Design review of the part built by this model. Coordinates are the model's own, in mm. Give positions to 0.01 mm unless a question says otherwise; leave off trailing zeros. Loops run counter-clockwise (first coordinate to the right, second up) from the corner with the lowest first, then second, coordinate; pieces in that order, holes last. Notation, with made-up numbers: (-19, -2) - (20, -2) arc R7 cw to (20, 5) - close; hole circle Ø3 at (40, -23). An arc over 180 degrees is marked (long way). Write each question's results on one line, items separated by ' | '.
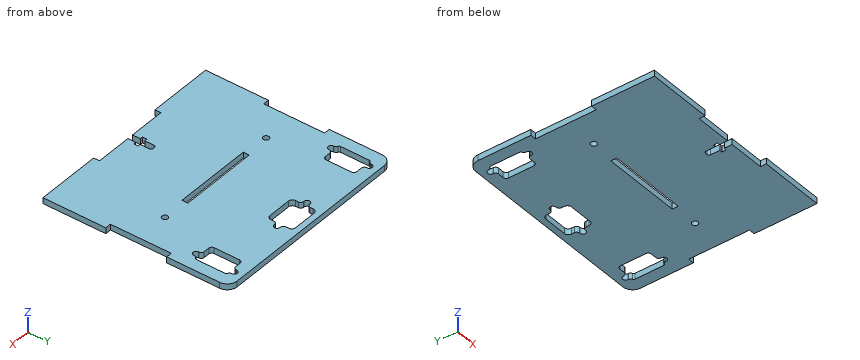
from build123d import *

# Parameters (mm, degrees)
ESBO_O1_W                = 100
ESBO_O1_H                = 95
RESSALTO_EXTRUS_O1_DEPTH = 1.5
ESBO_O2_R                = 1.5
ESBO_O2_W                = 40
ESBO_O2_H                = 3
CORTE_EXTRUS_O1_DEPTH    = 70.030790232
ESBO_O3_W                = 3
ESBO_O3_H                = 32
RESSALTO_EXTRUS_O2_DEPTH = 3
CUT_EXTRUDE1_DEPTH       = 72.233770081
CUT_EXTRUDE1_DEPTH_BACK  = 72.233770081
CUT_EXTRUDE4_DEPTH       = 72.186375101
CUT_EXTRUDE4_DEPTH_BACK  = 72.186375101
FILLET1_R                = 5


with BuildPart() as part:
    # Esboço1 → Ressalto-extrusão1 (new, symmetric)
    with BuildSketch(Plane.XY):
        Rectangle(ESBO_O1_W, ESBO_O1_H)
    extrude(amount=RESSALTO_EXTRUS_O1_DEPTH, both=True)

    # Esboço2 → Corte-extrusão1 (cut, through all)
    with BuildSketch(Plane.XY.offset(1.5)):
        with Locations((-33, -1)):
            Circle(ESBO_O2_R)
        with Locations(Location((33, -1, 0), (0, 0, 180))):
            Circle(ESBO_O2_R)
        with Locations((0, -46)):
            Rectangle(ESBO_O2_W, ESBO_O2_H)
        with Locations((0, -1)):
            Rectangle(ESBO_O2_W, ESBO_O2_H)
    extrude(amount=-CORTE_EXTRUS_O1_DEPTH, mode=Mode.SUBTRACT)

    # Esboço3 → Ressalto-extrusão2 (add, through all)
    with BuildSketch(Plane.XY.offset(1.5)):
        with Locations((-51.5, -31.5)):
            Rectangle(ESBO_O3_W, ESBO_O3_H)
        with Locations((51.5, -31.5)):
            Rectangle(ESBO_O3_W, ESBO_O3_H)
        with Locations((-51.5, 31.5)):
            Rectangle(ESBO_O3_W, ESBO_O3_H)
        with Locations((51.5, 31.5)):
            Rectangle(ESBO_O3_W, ESBO_O3_H)
    extrude(amount=-RESSALTO_EXTRUS_O2_DEPTH)

    # Sketch1 → Cut-Extrude1 (cut, two sides: drawn at the far end of the back side and taken through both)
    with BuildSketch(Plane(origin=(0, 0, -1.5), x_dir=(-1, 0, 0), z_dir=(0, 0, -1)).offset(-CUT_EXTRUDE1_DEPTH_BACK)):
        with BuildLine():
            Line((-36.5, 39.75), (-36.5, 26.75))
            ThreePointArc((-36.5, 26.75), (-36.939339828, 25.689339828), (-38, 25.25))
            Line((-38, 25.25), (-41, 25.25))
            ThreePointArc((-41, 25.25), (-42.060660172, 24.810660172), (-42.5, 23.75))
            Line((-42.5, 23.75), (-42.5, 23.5))
            ThreePointArc((-42.5, 23.5), (-44, 22), (-45.5, 23.5))
            Line((-45.5, 23.5), (-45.5, 23.75))
            ThreePointArc((-45.5, 23.75), (-45.74500996, 24.571583836), (-46.4, 25.124772708))
            ThreePointArc((-46.4, 25.124772708), (-46.836660027, 25.49356529), (-47, 26.041287847))
            Line((-47, 26.041287847), (-47, 40.458712153))
            ThreePointArc((-47, 40.458712153), (-46.836660027, 41.00643471), (-46.4, 41.375227292))
            ThreePointArc((-46.4, 41.375227292), (-45.74500996, 41.928416164), (-45.5, 42.75))
            Line((-45.5, 42.75), (-45.5, 43))
            ThreePointArc((-45.5, 43), (-44, 44.5), (-42.5, 43))
            Line((-42.5, 43), (-42.5, 42.75))
            ThreePointArc((-42.5, 42.75), (-42.060660172, 41.689339828), (-41, 41.25))
            Line((-41, 41.25), (-38, 41.25))
            ThreePointArc((-38, 41.25), (-36.939339828, 40.810660172), (-36.5, 39.75))
        make_face()
        with BuildLine():
            Line((-6, 44.5), (6, 44.5))
            ThreePointArc((6, 44.5), (7.414213562, 43.914213562), (8, 42.5))
            Line((8, 42.5), (8, 41))
            ThreePointArc((8, 41), (8.439339828, 39.939339828), (9.5, 39.5))
            Line((9.5, 39.5), (9.75, 39.5))
            ThreePointArc((9.75, 39.5), (11.25, 38), (9.75, 36.5))
            Line((9.75, 36.5), (9.5, 36.5))
            ThreePointArc((9.5, 36.5), (8.439339828, 36.060660172), (8, 35))
            Line((8, 35), (8, 33.5))
            ThreePointArc((8, 33.5), (7.414213562, 32.085786438), (6, 31.5))
            Line((6, 31.5), (-6, 31.5))
            ThreePointArc((-6, 31.5), (-7.414213562, 32.085786438), (-8, 33.5))
            Line((-8, 33.5), (-8, 35))
            ThreePointArc((-8, 35), (-8.439339828, 36.060660172), (-9.5, 36.5))
            Line((-9.5, 36.5), (-9.75, 36.5))
            ThreePointArc((-9.75, 36.5), (-11.25, 38), (-9.75, 39.5))
            Line((-9.75, 39.5), (-9.5, 39.5))
            ThreePointArc((-9.5, 39.5), (-8.439339828, 39.939339828), (-8, 41))
            Line((-8, 41), (-8, 42.5))
            ThreePointArc((-8, 42.5), (-7.414213562, 43.914213562), (-6, 44.5))
        make_face()
        with BuildLine():
            Line((47, 40.458712153), (47, 26.041287847))
            ThreePointArc((47, 26.041287847), (46.836660027, 25.49356529), (46.4, 25.124772708))
            ThreePointArc((46.4, 25.124772708), (45.74500996, 24.571583836), (45.5, 23.75))
            Line((45.5, 23.75), (45.5, 23.5))
            ThreePointArc((45.5, 23.5), (44, 22), (42.5, 23.5))
            Line((42.5, 23.5), (42.5, 23.75))
            ThreePointArc((42.5, 23.75), (42.060660172, 24.810660172), (41, 25.25))
            Line((41, 25.25), (38, 25.25))
            ThreePointArc((38, 25.25), (36.939339828, 25.689339828), (36.5, 26.75))
            Line((36.5, 26.75), (36.5, 39.75))
            ThreePointArc((36.5, 39.75), (36.939339828, 40.810660172), (38, 41.25))
            Line((38, 41.25), (41, 41.25))
            ThreePointArc((41, 41.25), (42.060660172, 41.689339828), (42.5, 42.75))
            Line((42.5, 42.75), (42.5, 43))
            ThreePointArc((42.5, 43), (44, 44.5), (45.5, 43))
            Line((45.5, 43), (45.5, 42.75))
            ThreePointArc((45.5, 42.75), (45.74500996, 41.928416164), (46.4, 41.375227292))
            ThreePointArc((46.4, 41.375227292), (46.836660027, 41.00643471), (47, 40.458712153))
        make_face()
    extrude(amount=CUT_EXTRUDE1_DEPTH + CUT_EXTRUDE1_DEPTH_BACK, mode=Mode.SUBTRACT)

    # Sketch2 → Cut-Extrude4 (cut, two sides: drawn at the far end of the back side and taken through both)
    with BuildSketch(Plane.XY.offset(-CUT_EXTRUDE4_DEPTH_BACK)):
        with BuildLine():
            Line((-0.5, -32.5), (0.5, -32.5))
            ThreePointArc((0.5, -32.5), (1.207106781, -32.792893219), (1.5, -33.5))
            Line((1.5, -33.5), (1.5, -38.23))
            Line((1.5, -38.23), (2.85, -38.23))
            Line((2.85, -38.23), (2.85, -40.5))
            Line((2.85, -40.5), (1.5, -40.5))
            Line((1.5, -40.5), (1.5, -44.5))
            Line((1.5, -44.5), (-1.5, -44.5))
            Line((-1.5, -44.5), (-1.5, -40.5))
            Line((-1.5, -40.5), (-2.85, -40.5))
            Line((-2.85, -40.5), (-2.85, -38.23))
            Line((-2.85, -38.23), (-1.5, -38.23))
            Line((-1.5, -38.23), (-1.5, -33.5))
            ThreePointArc((-1.5, -33.5), (-1.207106781, -32.792893219), (-0.5, -32.5))
        make_face()
    extrude(amount=CUT_EXTRUDE4_DEPTH + CUT_EXTRUDE4_DEPTH_BACK, mode=Mode.SUBTRACT)

    # Fillet1
    fillet1_edges = [part.edges().sort_by_distance(p)[0] for p in [
        (53, 47.5, 0),
        (-53, 47.5, 0),
    ]]
    fillet(fillet1_edges, radius=FILLET1_R)


solid = part.part
(1) Take a section at D-D on x = 15.5. Give the boundary of the cut face in (y, z), plus the area to 3 significant figures.
Answers below:
outline: (-44.5, -1.5) - (-2.5, -1.5) - (-2.5, 1.5) - (-44.5, 1.5) - close; (0.5, -1.5) - (47.5, -1.5) - (47.5, 1.5) - (0.5, 1.5) - close | area: 267 mm2
(2) Take a section at C-C on y = 13.5. Give the boundary of the cut face in (x, z), plus the area to 3 significant figures.
Answers below:
outline: (-50, -1.5) - (50, -1.5) - (50, 1.5) - (-50, 1.5) - close | area: 300 mm2
(3) Take a section at B-B on z = 0.2. Count the separate pieces of the cut face and the enclosed holes in it, plus the area to 3 significant figures.
Answers below:
separate pieces: 1 | enclosed holes: 6 | area: 8,980 mm2
(4) Take a section at A-A on x = 44. Give the boundary of the cut face in (y, z).
Answers below:
outline: (-47.5, -1.5) - (22, -1.5) - (22, 1.5) - (-47.5, 1.5) - close; (44.5, -1.5) - (47.5, -1.5) - (47.5, 1.5) - (44.5, 1.5) - close
(5) Wall thickness on line 1 along Y through (x, z) = (4, 0.45); line 2 along Y through (x, z) = (-0.5, -1.05); line 3 along Y through (x, z) = (33, -0.1): over which ranges is each line inside the solid? List them lowest first. Write a range as from..to.
Answers below:
line 1: -44.5..-2.5, 0.5..31.5, 44.5..47.5 | line 2: -32.5..-2.5, 0.5..31.5, 44.5..47.5 | line 3: -47.5..-2.5, 0.5..47.5
(6) Insertion check: P1, Ø0.9, axis at y = 3.5, z = 0.5, coming from the +X side; P2, Ø1.5, axis at x = -2, z = -0.5, coming from the -Y side. Each pin has a flat end and moves straight along its axis. Give the tip position at first contact, or say it passes through.
Answers below:
P1: x = 50 | P2: y = -44.5
